```python
from build123d import *

# Parameters (mm, degrees)
SKETCH3_W               = 110
SKETCH3_H               = 3.5
SKETCH4_R               = 0.95
BOSS_EXTRUDE2_DEPTH     = 2.5
MIRROR4_COPY_1_SKETCH_R = 0.95
MIRROR4_COPY_1_DEPTH    = 2.5
CUT_EXTRUDE1_REACH      = 99.4
SKETCH5_W               = 90
SKETCH5_H               = 110
SKETCH6_W               = 70
SKETCH6_H               = 90
CUT_EXTRUDE2_DEPTH      = 138.4
SKETCH7_R               = 0.925
CUT_EXTRUDE3_DEPTH      = 98.4
SKETCH9_R               = 0.925
CUT_EXTRUDE5_DEPTH      = 138.4
SKETCH8_W               = 76
SKETCH8_H               = 1
SKETCH8_W_2             = 1
SKETCH8_H_2             = 116
CUT_EXTRUDE4_DEPTH      = 103


with BuildPart() as part:
    # Sweep1: sweep along a path in Sketch1
    with BuildLine(Plane.XY) as sweep1_path:
        Line((45, -60), (45, 60))
        ThreePointArc((45, 60), (43.535533906, 63.535533906), (40, 65))
        Line((40, 65), (-40, 65))
        ThreePointArc((-40, 65), (-43.535533906, 63.535533906), (-45, 60))
        Line((-45, 60), (-45, -60))
        ThreePointArc((-45, -60), (-43.535533906, -63.535533906), (-40, -65))
        Line((-40, -65), (40, -65))
        ThreePointArc((40, -65), (43.535533906, -63.535533906), (45, -60))
    # Sketch3 → Sweep1 (sweep)
    with BuildSketch(Plane(origin=(40, 65, 0), x_dir=(0, 0, 1), z_dir=(-1, 0, 0))):
        with Locations((-52.5, 1.95)):
            Rectangle(SKETCH3_W, SKETCH3_H)
    sweep(path=sweep1_path.line)

    # Sketch4 → Boss-Extrude2 (add)
    with BuildSketch(Plane.XY.offset(2.5)):
        with BuildLine():
            Line((35.2, -65.2), (40, -65.2))
            ThreePointArc((40, -65.2), (43.676955262, -63.676955262), (45.2, -60))
            Line((45.2, -60), (45.2, -55.2))
            Line((45.2, -55.2), (38.2, -55.2))
            ThreePointArc((38.2, -55.2), (36.078679656, -56.078679656), (35.2, -58.2))
            Line((35.2, -58.2), (35.2, -65.2))
        make_face()
        with Locations((40, -60)):
            Circle(SKETCH4_R, mode=Mode.SUBTRACT)
    boss_extrude2 = extrude(amount=-BOSS_EXTRUDE2_DEPTH)

    # Mirror3: Boss-Extrude2 across plane
    add(boss_extrude2.mirror(Plane(origin=(0, 0, 0), x_dir=(0, 0, 1), z_dir=(1, 0, 0))))

    # Mirror4: Boss-Extrude2 across plane
    add(boss_extrude2.mirror(Plane.ZX))

    # Mirror4 copy 1 sketch → Mirror4 copy 1 (add)
    with BuildSketch(Plane(origin=(0, 0, 2.5), x_dir=(-1, 0, 0), z_dir=(0, 0, 1))):
        with BuildLine():
            Line((35.2, -65.2), (40, -65.2))
            ThreePointArc((40, -65.2), (43.676955262, -63.676955262), (45.2, -60))
            Line((45.2, -60), (45.2, -55.2))
            Line((45.2, -55.2), (38.2, -55.2))
            ThreePointArc((38.2, -55.2), (36.078679656, -56.078679656), (35.2, -58.2))
            Line((35.2, -58.2), (35.2, -65.2))
        make_face()
        with Locations((40, -60)):
            Circle(MIRROR4_COPY_1_SKETCH_R, mode=Mode.SUBTRACT)
    extrude(amount=-MIRROR4_COPY_1_DEPTH)

    # Sketch5 → Cut-Extrude1 (cut, up to next)
    with BuildSketch(Plane(origin=(48.7, 0, 0), x_dir=(0, 0, -1), z_dir=(1, 0, 0)), mode=Mode.PRIVATE) as cut_extrude1_sk1:
        with Locations((52.5, 0)):
            Rectangle(SKETCH5_W, SKETCH5_H)
    cut_extrude1_tool1 = extrude(cut_extrude1_sk1.sketch, amount=-CUT_EXTRUDE1_REACH, mode=Mode.PRIVATE) & part.part
    add(cut_extrude1_tool1.solids().sort_by_distance((48.7, 0, -52.5))[0], mode=Mode.SUBTRACT)

    # Sketch6 → Cut-Extrude2 (cut, through all)
    with BuildSketch(Plane(origin=(0, 68.7, 0), x_dir=(1, 0, 0), z_dir=(0, 1, 0))):
        with Locations((0, 52.5)):
            Rectangle(SKETCH6_W, SKETCH6_H)
    extrude(amount=-CUT_EXTRUDE2_DEPTH, mode=Mode.SUBTRACT)

    # Sketch7 → Cut-Extrude3 (cut, through all)
    with BuildSketch(Plane(origin=(48.7, 0, 0), x_dir=(0, 0, -1), z_dir=(1, 0, 0))):
        with Locations((102.5, 45)):
            Circle(SKETCH7_R)
        with Locations((102.5, -45)):
            Circle(SKETCH7_R)
    extrude(amount=-CUT_EXTRUDE3_DEPTH, mode=Mode.SUBTRACT)

    # Sketch9 → Cut-Extrude5 (cut, through all)
    with BuildSketch(Plane(origin=(0, 68.7, 0), x_dir=(1, 0, 0), z_dir=(0, 1, 0))):
        with Locations((-25, 102.5)):
            Circle(SKETCH9_R)
        with Locations((25, 102.5)):
            Circle(SKETCH9_R)
    extrude(amount=-CUT_EXTRUDE5_DEPTH, mode=Mode.SUBTRACT)

    # Sketch8 → Cut-Extrude4 (cut)
    with BuildSketch(Plane(origin=(0, 0, -107.5), x_dir=(-1, 0, 0), z_dir=(0, 0, -1))):
        with Locations((0, 67.2)):
            Rectangle(SKETCH8_W, SKETCH8_H)
        with Locations((-47.2, 0)):
            Rectangle(SKETCH8_W_2, SKETCH8_H_2)
        with Locations((0, -67.2)):
            Rectangle(SKETCH8_W, SKETCH8_H)
    extrude(amount=-CUT_EXTRUDE4_DEPTH, mode=Mode.SUBTRACT)


solid = part.part
```
Read the model definition and answer for the solid it produces. Units are mm, in the model's axes. A direction names the side the tool comes from. Give positions to 0.01 mm unless a question says otherwise; leave off trailing zeros. Order: outer loops, then holes, each group sorted by start corner. A loop starts at its lowest first (then second) coordinate and runs counter-clockwise, first axis right, second up. Notation, with made-up numbers: (9, 7) -> (49, 7) arc R10 cw to (49, 22) -> close; hole circle Ø5 at (10.5, 35). An arc over 180 degrees is marked (long way). Write item = value, one per line.
1. The mould has two halves that part along X. Classify faces 1 (the face through (-45.2, -1, -53)), 2 (the face through (-46.084, 66.219, -53.27)), 3 (the face through (46.084, -66.219, -53.27)), 4 (the face through (-43.717, -63.636, -52.998)): +X half, -X half, draft (parallel to the pull), parting line (faces both ways), or undercut.
Numbers:
face_1 = undercut
face_2 = -X half
face_3 = +X half
face_4 = undercut
2. Given pin 1 (0.8 mm diameter, centred on x = 48, z = -35.5, fed in from -Y), flat-ended and moving along its own axis, determine where the tip first touches the part or whether it passes through.
Numbers:
pin_1 = -64.23
3. A cutting plane is placed at B-B, the plane y = 15. Write down the section's boundary in (x, z), and give its area (3 significant figures).
Numbers:
outline = (-48.7, -107.5) -> (-45.2, -107.5) -> (-45.2, 2.5) -> (-48.7, 2.5) -> close; (45.2, -107.5) -> (46.7, -107.5) -> (46.7, -97.5) -> (45.2, -97.5) -> close; (45.2, -7.5) -> (46.7, -7.5) -> (46.7, -4.5) -> (47.7, -4.5) -> (47.7, -7.5) -> (48.7, -7.5) -> (48.7, 2.5) -> (45.2, 2.5) -> close; (47.7, -107.5) -> (48.7, -107.5) -> (48.7, -97.5) -> (47.7, -97.5) -> close
area = 442 mm²
4. A cutting plane is placed at A-A, the plane x = 6.5. Count the separate pieces of the cut face and the enclosed holes in it, and give its area (3 significant figures).
Numbers:
separate_pieces = 6
enclosed_holes = 0
area = 114 mm²
5. For faces 5 (the face through (-48.7, -1, -52)), 6 (the face through (-40.1, -61.2, 0)), determine the directions among +Z, -Z, +X, -X, +Y, -Y from which every point of the face is accessible in a straight line to the end or side of a thin tool.
Numbers:
face_5 = +Z, -Z, -X, +Y, -Y
face_6 = -Z
6. Straight lines are drawn through the part: line 1 along Z through (x, y) = (25, -68) (3 decimals); line 2 along X through (y, z) = (57.5, -10.5); line 3 along Y through (x, z) = (-30, -6). For each, find the intervals that lie inside material, in ascending order.
Numbers:
line_1 = -107.5 to -103.425, -101.575 to -97.5, -7.5 to 2.5
line_2 = -48.7 to -45.2, 45.2 to 46.7, 47.7 to 48.7
line_3 = -68.7 to -67.7, -66.7 to -65.2, 65.2 to 66.7, 67.7 to 68.7
